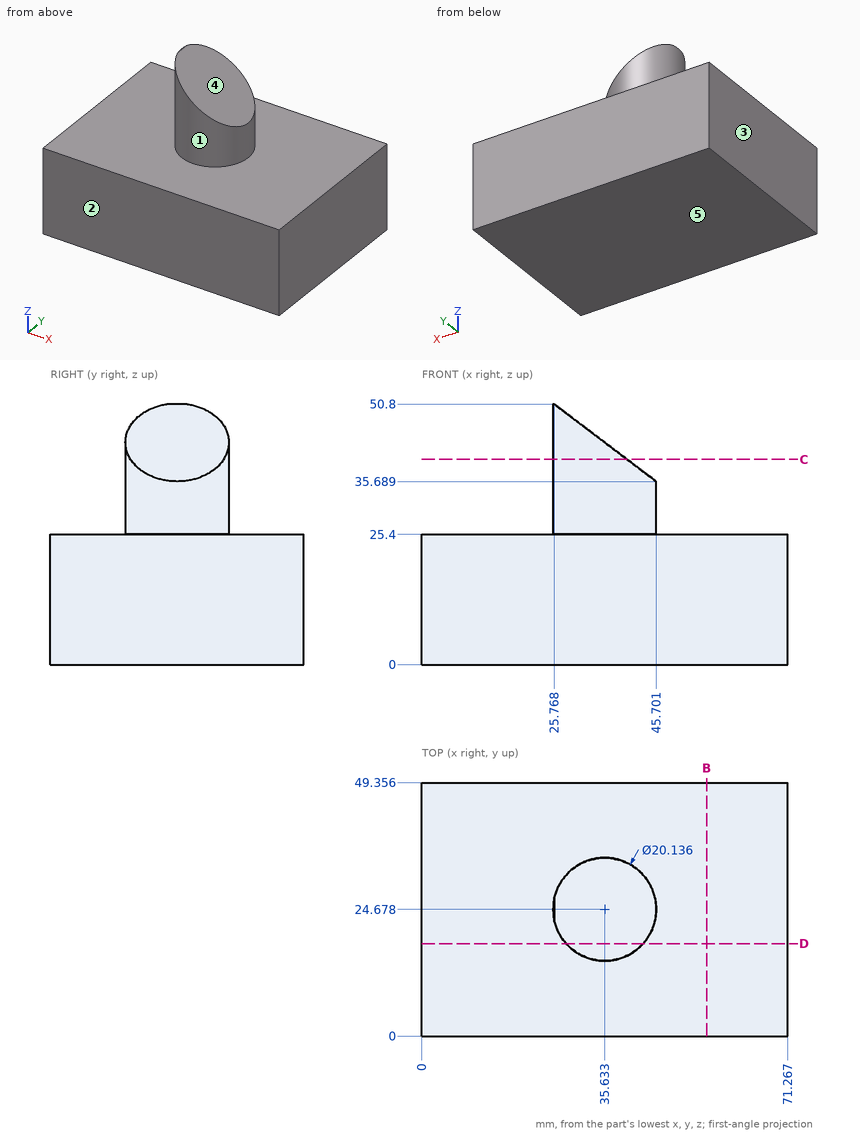
Drawing for the job (mm, zero at the part's lowest x, y, z). A direction names the side the tool comes from. Coordinates: 2 decimals unless noted, no trailing zeros. Write each loop counter-clockwise with the first axis right and the second up, starting at its lowest first coordinate (ties: lowest second). Pieces come first, ordered by that corner, then holes. Notation, with made-up numbers: (0.5, 37.25) - (25.5, 37.25) arc R26 cw to (25.5, 69.25) - close; hole circle Ø7 at (46, 10.25). An arc over 180 degrees is marked (long way). Write each question's results on one line, items separated by ' | '. Start each with the question number.
1) Cut at C-C (z = 40). Write the cut outline in (x, y) (1 decimal).
2) Mould opens along Z. For the marked faces 3, 4 and 5 say: pulls with the +Z half, pulls with the -Z half, needs draft (parallel to the pull), parting line crosses it, or undercut.
3) Probe line 1 along Z through (x, y) = (11, 25); line 2 along X through (y, z) = (20, 28); line 3 along Z through (x, y) = (36, 29) (1 decimal). List the from-to ranges inside material, lowest first. Write a range as from..to.
4) 3-axis set-ups, long thin cutter, end or side, ignore diameter. For the marked faces 1 and 2: which of +Z, -Z, +X, -X, +Y, -Y reach the whole face in a straight line?
5) Cut at B-B (x = 55.5). Write the cut outline in (y, z).
6) Cut at D-D (y = 18). Write the cut outline in (x, z).
7) Flat gauge pins, fed straight in: P1, Ø12, axis at x = 39, y = 30.5, coming from the +Z side; P2, Ø1, axis at x = 40, y = 19.5, coming from the +Z side; P3, Ø10, axis at y = 37, z = 44, coming from the -X side; P4, Ø8, axis at y = 7, z = 7.5, coming from the -X side. Where does each tip first touch, or does it go through?
Returned:
1) outline: (40, 15.6) - (40, 33.7) arc R10.1 ccw (long way) to start
2) face 3: needs draft | face 4: pulls with the +Z half | face 5: pulls with the -Z half
3) line 1: 0..25.4 | line 2: 26.72..44.55 | line 3: 0..43
4) face 1: +Z | face 2: +Z, -Z, +X, -X, -Y
5) outline: (0, 0) - (49.36, 0) - (49.36, 25.4) - (0, 25.4) - close
6) outline: (0, 0) - (71.27, 0) - (71.27, 25.4) - (43.17, 25.4) - (43.17, 37.61) - (28.1, 49.03) - (28.1, 25.4) - (0, 25.4) - close
7) P1: z = 45.32 | P2: z = 40.39 | P3: x = 28.72 | P4: x = 0
